Geometry: see drawing. Coordinates: mm, zero at the bounding-box minimum. Coordinates: 2 decimals unless noted, no trailing zeros. Loops run counter-clockwise (first coordinate to the right, second up) from the corner with the lowest first, then second, coordinate; pieces in that order, holes last. Notation, with made-up numbers: (36.5, -17.75) - (58.5, -17.75) arc R25 cw to (58.5, -1.75) - close; hole circle Ø4 at (29.5, 24). An arc over 180 degrees is marked (long way). Write each question's results on one line, items separated by ' | '. Start each with the question number.
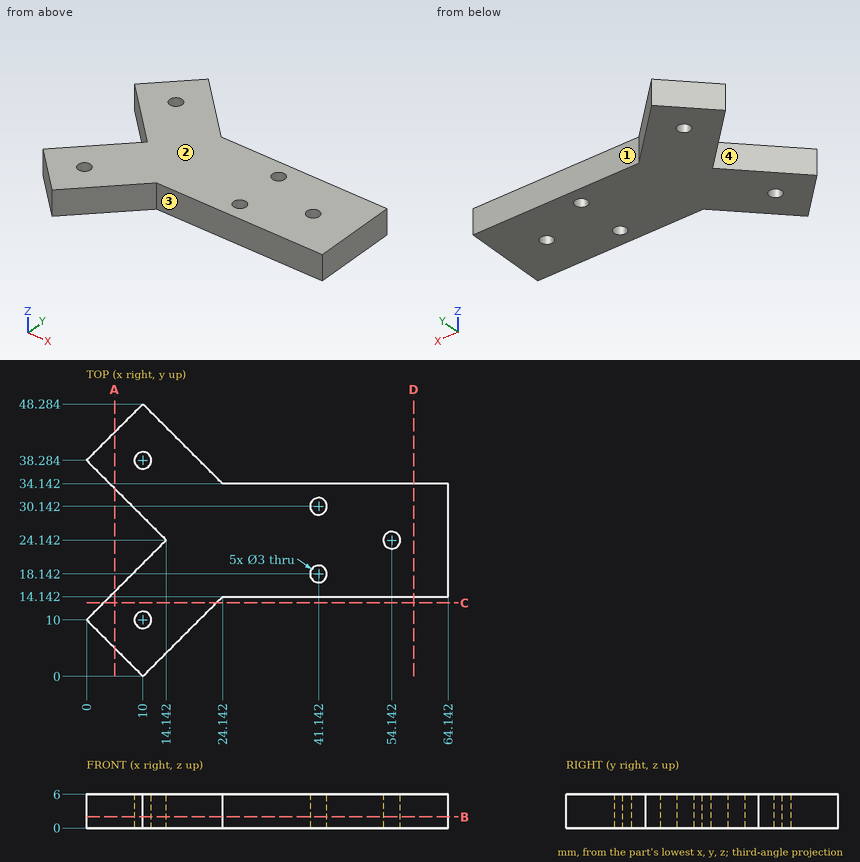
1) Section query C-C on y = 13. Output: boundary loops of the cut face in (x, z).
2) Material intervals for line 1 (Y direction, x = 41, z = 2.45) (1 decimal); line 2 (Y direction, x = 42, z = 4.7); line 3 (Y direction, x = 37, z = 1.9), sorted ascending. Write a range as [from, to].
3) Pull-direction query (Y, two-part tool) for the marked faces 1, 2, 3 and 4; classes: released by +Y, released by -Y, zero draft, split by the parting line, or undercut.
4) Section query A-A on x = 5. Output: boundary loops of the cut face in (y, z), and give its area (3 significant figures).
5) Pin query (flat end, axial travel): pin 1 Ø1.8 at (x, y) = (54.14, 24.14) entering from -Z; pin 2 Ø1.5 at (x, z) = (34.5, 2.5) entering from +Y. Return the tip coordinate at first contact, or that it passes through.
6) Section query B-B on z = 2. Output: boundary loops of the cut face in (x, y).
7) Section query D-D on x = 58. Output: boundary loops of the cut face in (y, z).
Returned:
1) outline: (3, 0) - (23, 0) - (23, 6) - (3, 6) - close
2) line 1: y = [14.1, 16.6], [19.6, 28.6], [31.6, 34.1] | line 2: y = [14.14, 16.91], [19.37, 28.91], [31.37, 34.14] | line 3: y = [14.14, 34.14]
3) face 1: released by +Y | face 2: zero draft | face 3: released by -Y | face 4: undercut
4) outline: (5, 0) - (15, 0) - (15, 6) - (5, 6) - close; (33.28, 0) - (43.28, 0) - (43.28, 6) - (33.28, 6) - close | area: 120 mm²
5) pin 1: passes through | pin 2: stops at y = 34.14
6) outline: (0, 10) - (10, 0) - (24.14, 14.14) - (64.14, 14.14) - (64.14, 34.14) - (24.14, 34.14) - (10, 48.28) - (0, 38.28) - (14.14, 24.14) - close; hole circle Ø3 at (10, 10); hole circle Ø3 at (10, 38.28); hole circle Ø3 at (41.14, 18.14); hole circle Ø3 at (41.14, 30.14); hole circle Ø3 at (54.14, 24.14)
7) outline: (14.14, 0) - (34.14, 0) - (34.14, 6) - (14.14, 6) - close
